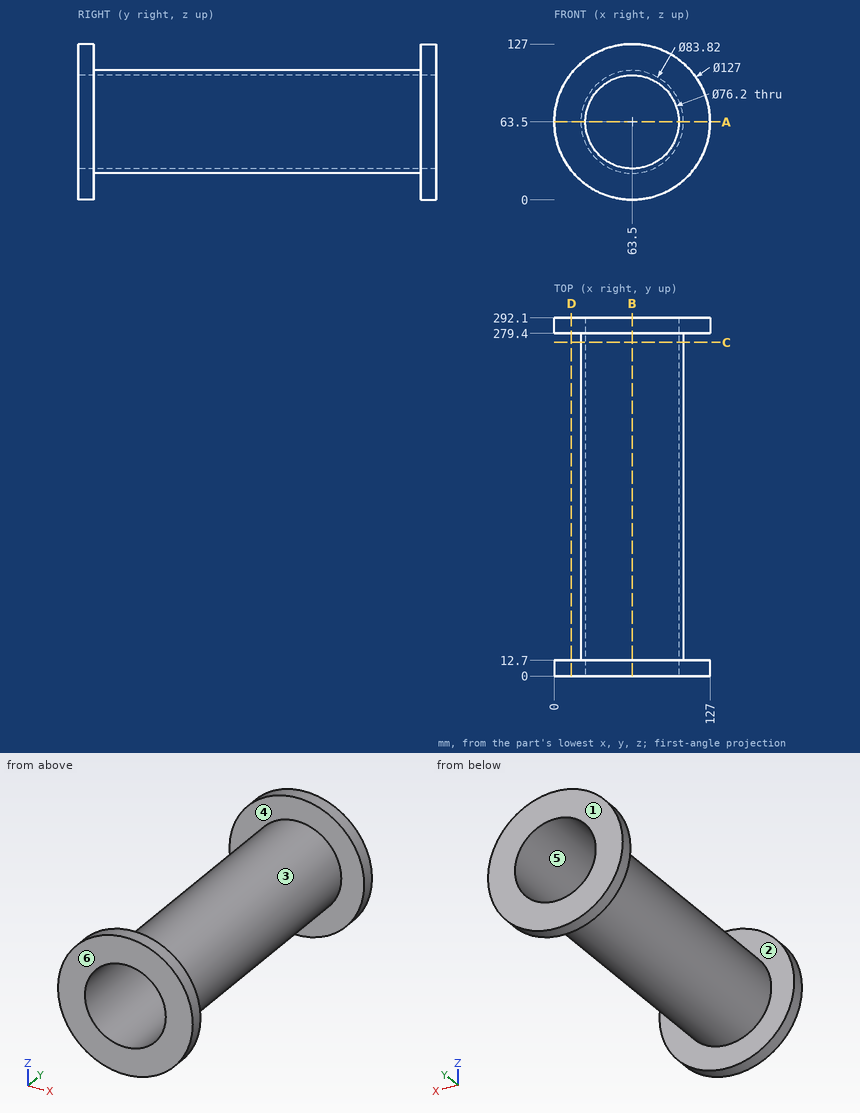
Source: three-view drawing plus pictorial views. Frame: mm from the lowest corner of the part. A direction names the side the tool comes from. Give positions to 0.01 mm unless a question says otherwise; leave off trailing zeros. Order: outer loops, then holes, each group sorted by start corner. A loop starts at its lowest first (then second) coordinate and runs counter-clockwise, first axis right, second up. Notation, with made-up numbers: M -1.5,60.5 L 14.5,60.5 A30 cw 14.5,83.5 Z; hole C -32.75,-37.5 d2. An arc over 180 degrees is marked long. One line per question, with ' | ' between items. Start each with the question number.
1. Material intervals for probe 1 along Y at (x, z) = (27, 37); probe 2 along X at (y, z) = (72, 63), sorted ascending. Write a range as [from, to].
2. Section query D-D (x = 14). Return the cut outline in (y, z).
3. Access query for the marked faces 1 and 2. Directions: +Z, -Z, +X, -X, +Y, -Y. A direction counts if a zero-diameter tool reaches every point of the face in a straight line with its end or side. Return the directions, or none.
4. Section query A-A (z = 63.5). Return the cut outline in (x, y).
5. Section query B-B (x = 63.5). Return the cut outline in (y, z).
6. Section query C-C (y = 272). Return the cut outline in (x, z), and give its area (3 significant figures).
7. Pull-direction query (Y, two-part tool) for the marked faces 3, 4, 5 and 6; classes: released by +Y, released by -Y, zero draft, split by the parting line, or undercut.
8. First-contact query: pin 1 Ø4 at (y, z) = (175.5, 70.5) entering from -X; pin 2 Ø3 at (x, y) = (95.5, 137) entering from +Z; pin 3 Ø10 at (y, z) = (207, 95.5) entering from +X; pin 4 Ø1 at (x, z) = (22, 54) entering from -Y. Flat tips, straight axial feed; report the tip coordinate or a pass-through.
Here are the results:
1) probe 1: [0, 12.7], [279.4, 292.1] | probe 2: [21.59, 25.4], [101.6, 105.41]
2) outline: M 0,23.73 L 12.7,23.73 L 12.7,103.27 L 0,103.27 Z; M 279.4,23.73 L 292.1,23.73 L 292.1,103.27 L 279.4,103.27 Z
3) face 1: +Z, -Z, +X, -X, +Y | face 2: none
4) outline: M 0,0 L 25.4,0 L 25.4,292.1 L 0,292.1 L 0,279.4 L 21.59,279.4 L 21.59,12.7 L 0,12.7 Z; M 101.6,0 L 127,0 L 127,12.7 L 105.41,12.7 L 105.41,279.4 L 127,279.4 L 127,292.1 L 101.6,292.1 Z
5) outline: M 0,0 L 12.7,0 L 12.7,21.59 L 279.4,21.59 L 279.4,0 L 292.1,0 L 292.1,25.4 L 0,25.4 Z; M 0,101.6 L 292.1,101.6 L 292.1,127 L 279.4,127 L 279.4,105.41 L 12.7,105.41 L 12.7,127 L 0,127 Z
6) outline: C 63.5,63.5 d83.82; hole C 63.5,63.5 d76.2 | area: 958 mm²
7) face 3: undercut | face 4: undercut | face 5: zero draft | face 6: released by -Y
8) pin 1: x = 21.89 | pin 2: z = 92.24 | pin 3: x = 95.55 | pin 4: y = 0
